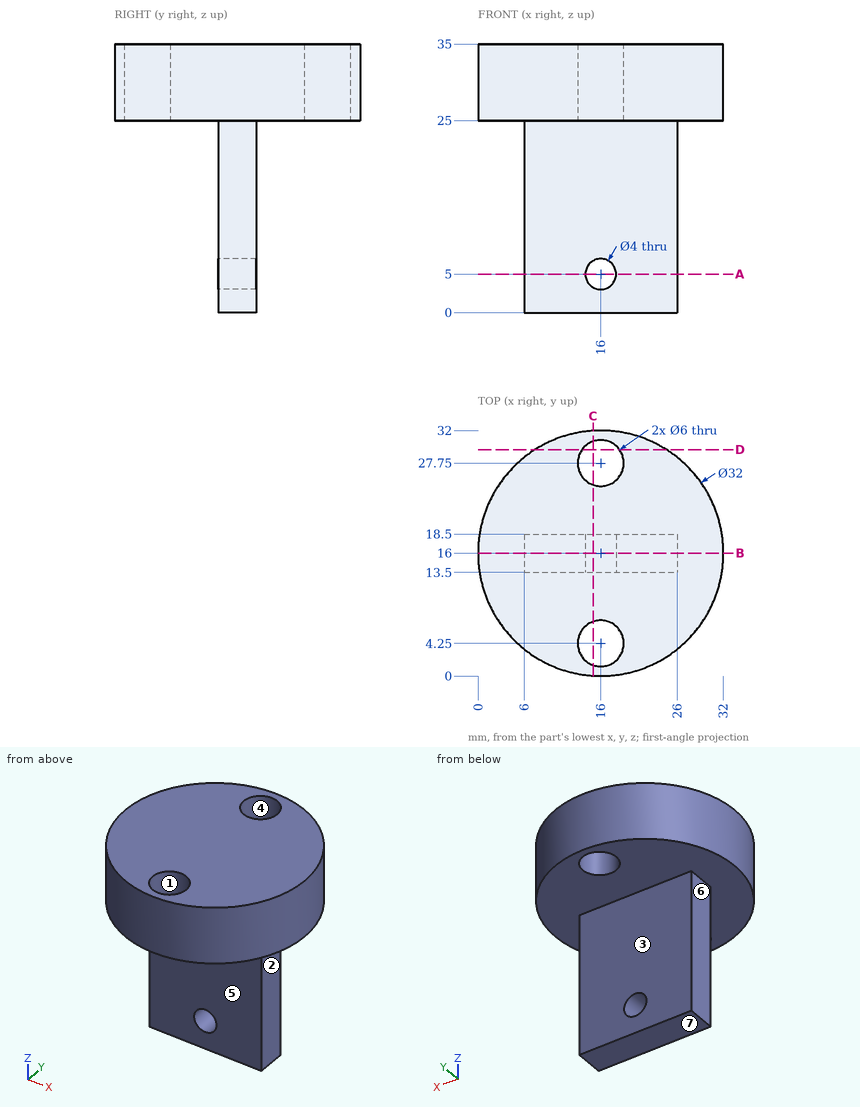
The figure shows three views and two pictorial views of one solid part (mm, origin at its lowest corner). Answer the questions. A direction names the side the tool comes from. Round coordinates to 2 decimals unless told otherwise and drop trailing zeros. Order: outer loops, then holes, each group sorted by start corner. A loop starts at its lowest first (then second) coordinate and runs counter-clockwise, first axis right, second up.
Q1. Given pin 1 Ø12 at (x, z) = (19.5, 10.5) entering from -Y; pin 2 Ø10 at (y, z) = (10.5, 31.5) entering from -X; pin 3 Ø1.5 at (x, y) = (13, 20) entering from -Z; pin 4 Ø4 at (y, z) = (22, 11.5) entering from +X, each flat-ended and moving along its own axis, determine where each tip first touches the part or whether it passes through.
Solution:
pin 1: stops at y = 13.5
pin 2: stops at x = 0.01
pin 3: stops at z = 25
pin 4: passes through
Q2. A cutting plane is placed at C-C, the plane x = 15. Determine the outline of the cut face in (y, z), then the cut area to 3 significant figures.
Solution:
outline: (0.03, 25) - (1.42, 25) - (1.42, 35) - (0.03, 35) - close; (7.08, 25) - (13.5, 25) - (13.5, 6.73) - (18.5, 6.73) - (18.5, 25) - (24.92, 25) - (24.92, 35) - (7.08, 35) - close; (13.5, 0) - (18.5, 0) - (18.5, 3.27) - (13.5, 3.27) - close; (30.58, 25) - (31.97, 25) - (31.97, 35) - (30.58, 35) - close
area: 314 mm2
Q3. The mould has two halves that part along Y. Classify the marked faces 1, 2, 3 and 4: pulls with the +Y half, pulls with the -Y half, needs draft (parallel to the pull), parting line crosses it, or undercut.
Solution:
face 1: undercut
face 2: needs draft
face 3: pulls with the +Y half
face 4: undercut
Q4. A cutting plane is placed at B-B, the plane y = 16. Determine the outline of the cut face in (x, z).
Solution:
outline: (0, 25) - (6, 25) - (6, 0) - (26, 0) - (26, 25) - (32, 25) - (32, 35) - (0, 35) - close; hole circle Ø4 at (16, 5)
Q5. A cutting plane is placed at D-D, the plane y = 29.5. Determine the outline of the cut face in (x, z), then the cut area to 3 significant figures.
Solution:
outline: (7.41, 25) - (13.56, 25) - (13.56, 35) - (7.41, 35) - close; (18.44, 25) - (24.59, 25) - (24.59, 35) - (18.44, 35) - close
area: 123 mm2
Q6. A tool of negligible diameter and unlimited length cuts with its end or side. For the marked faces 5, 6 and 7, from which of +Z, -Z, +X, -X, +Y, -Y can it reach the whole face along a straight path? Write none if from no direction.
Solution:
face 5: -Z, +X, -X, -Y
face 6: -Z, -X, +Y, -Y
face 7: -Z, +X, -X, +Y, -Y
Q7. A cutting plane is placed at A-A, the plane z = 5. Determine the outline of the cut face in (x, y).
Solution:
outline: (6, 13.5) - (14, 13.5) - (14, 18.5) - (6, 18.5) - close; (18, 13.5) - (26, 13.5) - (26, 18.5) - (18, 18.5) - close
Q8. Find the intervals of material crossed by line 1 along Y through (x, z) = (16, 31); line 2 along Y through (x, z) = (14.5, 33.5); line 3 along Z through (x, y) = (20.5, 12), in increasing order.
Solution:
line 1: y = 0 to 1.25, 7.25 to 24.75, 30.75 to 32
line 2: y = 0.07 to 1.65, 6.85 to 25.15, 30.35 to 31.93
line 3: z = 25 to 35
